from build123d import *

# Parameters (mm, degrees)
BOSS_EXTRUDE1_DEPTH = 7
FILLET1_START       = -25
FILLET1_DEPTH       = 50
FILLET2_RADIUS      = 3.5
FILLET2_LENGTH      = 38.000003375


with BuildPart() as part:
    # Sketch1 → Boss-Extrude1 (new body)
    with BuildSketch(Plane(origin=(0, 0, 0), x_dir=(1, 0, 0), z_dir=(0, 1, 0))):
        with BuildLine():
            Line((137.927515414, 24.000010242), (175, 24.000010242))
            Line((175, 24.000010242), (175, -24))
            Line((175, -24), (137.927515472, -24.000009912))
            ThreePointArc((137.927515472, -24.000009912), (138.338710325, -21.50351659), (138.704722342, -19))
            Line((138.704722342, -19), (165, -19))
            Line((165, -19), (165, 19.000003375))
            Line((165, 19.000003375), (138.70472188, 19.000003375))
            ThreePointArc((138.70472188, 19.000003375), (138.338710037, 21.503518438), (137.927515414, 24.000010242))
        make_face()
    extrude(amount=BOSS_EXTRUDE1_DEPTH)

    # Fillet1: read off the stored shape, not the designer's step
    # Fillet1 outline → Fillet1 (cut)
    with BuildSketch(Plane.XY.offset(FILLET1_START)):
        with BuildLine():
            ThreePointArc((171.5, 7), (173.974873734, 5.974873734), (175, 3.5))
            Line((175, 3.5), (175, 7))
            Line((175, 7), (171.5, 7))
        make_face()
        with BuildLine():
            ThreePointArc((175, 3.5), (173.974873734, 1.025126266), (171.5, 0))
            Line((171.5, 0), (175, 0))
            Line((175, 0), (175, 3.5))
        make_face()
    extrude(amount=FILLET1_DEPTH, mode=Mode.SUBTRACT)

    # Fillet2: full round fillet: the end face becomes a half cylinder, R = half its width
    fillet2_face = Plane((165, 3.5, -1.687e-06), x_dir=(0, 0, 1), z_dir=(-1, 0, 0))  # on the end face: x along it, z out of the body
    fillet2_slab = fillet2_face.offset(-FILLET2_RADIUS / 2) * Box(FILLET2_LENGTH, 2 * FILLET2_RADIUS, FILLET2_RADIUS, mode=Mode.PRIVATE)  # the body's end, R deep
    fillet2_round = Plane((168.5, 3.5, -1.687e-06), x_dir=(-1, 0, 0), z_dir=(0, 0, 1)) * Cylinder(FILLET2_RADIUS, FILLET2_LENGTH, mode=Mode.PRIVATE)  # its axis R under the face
    add(fillet2_slab - fillet2_round, mode=Mode.SUBTRACT)


solid = part.part
Geometry: final body of the model. Coordinates: model frame, mm. A direction names the side the tool comes from. Give positions to 0.01 mm unless a question says otherwise; leave off trailing zeros. Write each loop counter-clockwise with the first axis right and the second up, starting at its lowest first coordinate (ties: lowest second). Pieces come first, ordered by that corner, then holes.
(1) Mould query, pull axis Z, two halves, no side actions, for faces 1 (the flat face through (156, 3, -24)), 2 (the flat face through (154, 3, -19)), 3 (the flat face through (157, 3, 24)). Classes: released by +Z, released by -Z, zero draft, split by the parting line, or undercut.
(2) Access query for faces 4 (the cylindrical face through (165, 3.6, 0.3)), 5 (the flat face through (170, 7, 0)), 6 (the cylindrical face through (138.333, 3.451, 21.539)). Directions: +Z, -Z, +X, -X, +Y, -Y. A direction counts if a zero-diameter tool reaches every point of the face in a straight line with its end or side. Return the directions, or none.
(3) Cut plane A-A, the plane x = 144.5. Return loops of the section in (y, z), then the cut area to 3 significant figures.
(4) First-contact query: P1, Ø1, axis at y = 5.5, z = -13, coming from the -X side; P2, Ø1, axis at x = 167, z = 12.5, coming from the +Y side. Flat tips, straight axial feed; report the tip coordinate or a pass-through.
(5) Cut plane B-B, the plane y = 6.5. Return loops of the section in (x, z).
(6) Cut plane D-D, the plane x = 166. Return loops of the section in (y, z).
(7) Ray query, line 1 (Z direction, x = 165.5, y = 0.75); line 2 (X direction, y = 2.75, z = -21); line 3 (X direction, y = 2.5, z = 10.5). Return the intervals inside material, ascending.
(8) Cut plane C-C, the plane z = -5.5. Return loops of the section in (x, y), then the cut area to 3 significant figures.
Values follow:
1. face 1: released by -Z
1. face 2: undercut
1. face 3: released by +Z
2. face 4: -X
2. face 5: +Z, -Z, +X, -X, +Y
2. face 6: -X, +Y, -Y
3. outline: (0, -24) - (7, -24) - (7, -19) - (0, -19) - close; (0, 19) - (7, 19) - (7, 24) - (0, 24) - close
3. area: 70.0 mm2
4. P1: stops at x = 165.34
4. P2: stops at y = 6.85
5. outline: (137.93, -24) - (173.3, -24) - (173.3, 24) - (137.93, 24) arc R140 cw to (138.7, 19) - (166.7, 19) - (166.7, -19) - (138.7, -19) arc R140 cw to start
6. outline: (0, -24) - (7, -24) - (7, -19) - (5.95, -19) - (5.95, 19) - (7, 19) - (7, 24) - (0, 24) - (0, 19) - (1.05, 19) - (1.05, -19) - (0, -19) - close
7. line 1: z = -24 to -19, 19 to 24
7. line 2: x = 138.42 to 174.92
7. line 3: x = 165.15 to 174.85
8. outline: (168.5, 0) - (171.5, 0) arc R3.5 ccw to (171.5, 7) - (168.5, 7) arc R3.5 ccw to start
8. area: 59.5 mm2
